from build123d import *

# Parameters (mm, degrees)
SKETCH1_R           = 20
BOSS_EXTRUDE1_DEPTH = 70
SKETCH2_R           = 4
BOSS_EXTRUDE2_DEPTH = 25
FILLET1_R           = 5


with BuildPart() as part:
    # Sketch1 → Boss-Extrude1 (new body)
    with BuildSketch(Plane.XY):
        Circle(SKETCH1_R)
    extrude(amount=BOSS_EXTRUDE1_DEPTH)

    # Sketch2 → Boss-Extrude2 (add)
    with BuildSketch(Plane.XY.offset(70)):
        Circle(SKETCH2_R)
    extrude(amount=BOSS_EXTRUDE2_DEPTH)

    # Fillet1
    fillet1_edges = [part.edges().sort_by_distance(p)[0] for p in [
        (-20, 0, 0),
        (-20, 0, 70),
    ]]
    fillet(fillet1_edges, radius=FILLET1_R)


solid = part.part
Geometry check sheet. Reference: the model listing, model coordinates, mm. A direction names the side the tool comes from. Give positions to 0.01 mm unless a question says otherwise; leave off trailing zeros. Write each loop counter-clockwise with the first axis right and the second up, starting at its lowest first coordinate (ties: lowest second). Pieces come first, ordered by that corner, then holes.
1) Cross-section at A-A (y = 0). Record the boundary of the cut face in (x, z), plus the area to 3 significant figures.
Values follow:
outline: (-20, 5) arc R5 ccw to (-15, 0) - (15, 0) arc R5 ccw to (20, 5) - (20, 65) arc R5 ccw to (15, 70) - (4, 70) - (4, 95) - (-4, 95) - (-4, 70) - (-15, 70) arc R5 ccw to (-20, 65) - close
area: 2,980 mm2
2) Thickness scan on line 1 (Z direction, x = 0, y = -5); line 2 (X direction, y = 0.5, z = 30.5); line 3 (Y direction, x = 7.5, z = 35.5). Record the ranges inside material, lowest first.
Values follow:
line 1: z = 0 to 70
line 2: x = -19.99 to 19.99
line 3: y = -18.54 to 18.54
3) Go/stop test with flat-tipped pins: pin 1 Ø5 at (x, z) = (13.5, 52.5) entering from -Y; pin 2 Ø2 at (x, y) = (-2.5, -14) entering from +Z; pin 3 Ø3 at (x, y) = (12, -12.5) entering from -Z. Record where each tip stops, or that it passes through.
Values follow:
pin 1: stops at y = -16.7
pin 2: stops at z = 70
pin 3: stops at z = 0.07
4) Set-up check for faces 1 (the face through (-4.336, -19.524, 34.58)), 2 (the face through (-0.867, -3.905, 82.325)): record each of +Z, -Z, +X, -X, +Y, -Y from which the full face is reachable in a straight line by a thin tool's end or side.
Values follow:
face 1: +Z, -Z
face 2: +Z
5) Cross-section at D-D (z = 68). Record the boundary of the cut face in (x, y), plus the area to 3 significant figures.
Values follow:
outline: circle Ø38 at (0, 0)
area: 1,130 mm2
6) Cross-section at C-C (z = 49). Record the boundary of the cut face in (x, y), plus the area to 3 significant figures.
Values follow:
outline: circle Ø40 at (0, 0)
area: 1,260 mm2
